Input: part model. Units: mm. Frame: model coordinates. Face numbers are marked on the shaded views. A direction names the side the tool comes from. Coordinates: 2 decimals unless noted, no trailing zeros. Order: outer loops, then holes, each group sorted by start corner. A loop starts at its lowest first (then second) coordinate and runs counter-clockwise, first axis right, second up. Notation, with made-up numbers: (77.5, 17) -> (133.5, 17) arc R19 ccw to (133.5, 47) -> close; hole circle Ø11 at (2.25, 51). An arc over 180 degrees is marked (long way). Use CSV: the item, a comma, the result in double quotes. Start each with the question number.
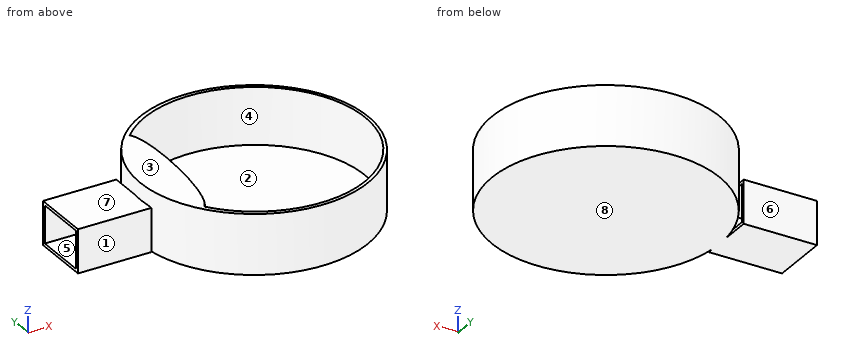
```python
from build123d import *

# Parameters (mm, degrees)
F0_W     = 49
F0_H     = 39
F1_DEPTH = 29
F3_R     = 76.2
F4_DEPTH = 40
F5_R     = 73.66
F6_DEPTH = 38
F2_W     = 35
F2_H     = 25
F7_DEPTH = 147.5
F9_DEPTH = 38


with BuildPart() as f1:
    # F0 (on Top) → F1 (new body)
    with BuildSketch(Plane.XY):
        with Locations((-50.2903954238, 2.6249693376)):
            Rectangle(F0_W, F0_H)
    extrude(amount=F1_DEPTH)

    # F3 (on Top) → F4 (join)
    with BuildSketch(Plane.XY):
        with Locations((50.0179536991, -5.090871723)):
            Circle(F3_R)
    extrude(amount=F4_DEPTH)

    # F5 (on face) → F6 (cut)
    with BuildSketch(Plane.XY.offset(40)):
        with Locations((50.5579536991, -5.090871723)):
            Circle(F5_R)
    extrude(amount=-F6_DEPTH, mode=Mode.SUBTRACT)

    # F2 (on face) → F7 (cut)
    with BuildSketch(Plane(origin=(-74.7903954238, 0, 0), x_dir=(0, -1, 0), z_dir=(-1, 0, 0))):
        with Locations((-2.6249693376, 14.5)):
            Rectangle(F2_W, F2_H)
    extrude(amount=-F7_DEPTH, mode=Mode.SUBTRACT)

    # F8 (on face) → F9 (join)
    with BuildSketch(Plane.XY.offset(2)):
        with BuildLine():
            ThreePointArc((-22.4493461678, -14.8750306624), (-17.8813273172, -32.3279863642), (-9.2079011268, -48.147093073))
            add(Edge.make_bspline(
                [(-2.5791042219, 45.9213687248), (6.562867427, 35.1885122385), (1.3712482781, -38.7284297831), (-9.2079011268, -48.147093073)],
                knots=[0.5957171177, 0.5957171177, 0.5957171177, 0.5957171177, 1, 1, 1, 1], degree=3))
            ThreePointArc((-2.5791042219, 45.9213687248), (-11.9603198587, 33.8611637996), (-18.6515612509, 20.1249693376))
            Line((-18.6515612509, 20.1249693376), (-21.8889399872, 20.1249693376))
            ThreePointArc((-21.8889399872, 20.1249693376), (-22.927932873, 16.9395080336), (-23.8258859148, 13.7114513007))
            add(Edge.make_bspline(
                [(-25.7903954238, -12.9307361878), (-26.0689147995, -8.6981558447), (-26.1124652464, 0.3286887969), (-24.7810032726, 9.273748372), (-23.8258859148, 13.7114513007)],
                knots=[0.2496191663, 0.2496191663, 0.2496191663, 0.2496191663, 0.2970853564, 0.3479233847, 0.3479233847, 0.3479233847, 0.3479233847], degree=3))
            Line((-25.7903954238, -12.9307361878), (-25.7903954238, -12.8067127836))
            ThreePointArc((-25.7903954238, -12.8067127836), (-25.6779062067, -13.8416884355), (-25.5512876221, -14.8750306624))
            Line((-25.5512876221, -14.8750306624), (-22.4493461678, -14.8750306624))
        make_face()
    extrude(amount=F9_DEPTH)


solid = f1.part
```
1. Material intervals for line 1 along Y through (x, z) = (-46, 16.5); line 2 along Z through (x, y) = (37.5, -74.5); line 3 along Y through (x, z) = (104, 19), sorted ascending.
2. Section D-D on x = 46. Return loops of the section in (y, z).
3. Pull-direction query (Y, two-part tool) for the marked faces 1, 2 and 3; classes: released by +Y, released by -Y, zero draft, split by the parting line, or undercut.
4. Section C-C on z = 16.5. State how many separate pieces and enclosed holes the cut face has, then the cut area to 3 significant figures.
5. Access query for the marked faces 4, 5, 6, 7 and 8. Directions: +Z, -Z, +X, -X, +Y, -Y. A direction counts if a zero-diameter tool reaches every point of the face in a straight line with its end or side. Return the directions, or none.
6. Section B-B on y = -71.5. Return loops of the section in (x, z), then the cut area to 3 significant figures.
7. Section A-A on x = -57. Return loops of the section in (y, z).
8. Contact query for flat-ended pins moving along their axis: P1, Ø19.5, axis at x = -61, y = -1.5, coming from the +Z side; P2, Ø2, axis at x = -13.5, z = 28.5, coming from the +Y side; P3, Ø12, axis at x = 81.5, y = -35.5, coming from the +Z side. Output: stop coordinate, or through.
Values follow:
1,line 1,"y = -16.88 to -14.88, 20.12 to 22.12"
1,line 2,"z = 0 to 2"
1,line 3,"y = -58.87 to -55.78, 45.6 to 48.69"
2,outline,"(-81.18, 0) -> (71, 0) -> (71, 40) -> (68.43, 40) -> (68.43, 2) -> (-78.61, 2) -> (-78.61, 40) -> (-81.18, 40) -> close"
3,face 1,"released by -Y"
3,face 2,"undercut"
3,face 3,"zero draft"
4,separate pieces,"3"
4,enclosed holes,"1"
4,area,"3,020 mm2"
5,face 4,"+Z"
5,face 5,"-X"
5,face 6,"+Z, -Z, -X, +Y"
5,face 7,"+Z, -X, +Y, -Y"
5,face 8,"-Z, +X, -X, +Y, -Y"
6,outline,"(12.65, 0) -> (87.38, 0) -> (87.38, 40) -> (82.43, 40) -> (82.43, 2) -> (18.69, 2) -> (18.69, 40) -> (12.65, 40) -> close"
6,area,"567 mm2"
7,outline,"(-16.88, 0) -> (22.12, 0) -> (22.12, 29) -> (-16.88, 29) -> close; hole (-14.88, 2) -> (20.12, 2) -> (20.12, 27) -> (-14.88, 27) -> close"
8,P1,"stops at z = 29"
8,P2,"stops at y = 38.47"
8,P3,"stops at z = 2"
